from build123d import *

# Parameters (mm, degrees)
SKETCH1_R           = 4
BOSS_EXTRUDE1_DEPTH = 3


with BuildPart() as part:
    # Sketch1 → Boss-Extrude1 (new body)
    with BuildSketch(Plane.XY):
        with BuildLine():
            Line((-3.41129842, 4.305994118), (3.41129842, -4.305994118))
            Line((3.41129842, -4.305994118), (7.005179011, -1.458846897))
            Line((7.005179011, -1.458846897), (8.621253306, -3.498775848))
            Line((8.621253306, -3.498775848), (11.505363509, -2.105535978))
            Line((11.505363509, -2.105535978), (23.000363507, -2.105335353))
            ThreePointArc((23.000363507, -2.105335353), (28.559669511, 3.611172521), (23.925659877, 10.100417487))
            Line((23.925659877, 10.100417487), (0.454659877, 10.100417487))
            Line((0.454659877, 10.100417487), (-0.813143143, 8.410019752))
            Line((-0.813143143, 8.410019752), (0.182582172, 7.153141338))
            Line((0.182582172, 7.153141338), (-3.41129842, 4.305994118))
        make_face()
        with Locations((23.217363507, 3.802664647)):
            Circle(SKETCH1_R, mode=Mode.SUBTRACT)
        Polygon((2.283340507, 4.456152944), (4.860365799, 1.203240304), (2.39128753, -0.752815038), (-0.185737762, 2.500097602), align=None, mode=Mode.SUBTRACT)
    extrude(amount=-BOSS_EXTRUDE1_DEPTH)


solid = part.part
Input: part model. Units: mm. Frame: model coordinates. A direction names the side the tool comes from. Round coordinates to 2 decimals unless told otherwise and drop trailing zeros. Order: outer loops, then holes, each group sorted by start corner. A loop starts at its lowest first (then second) coordinate and runs counter-clockwise, first axis right, second up. Notation, with made-up numbers: (30.25, 36) - (80.25, 36) arc R21 cw to (80.25, 73) - close; hole circle Ø2 at (84, 66). An arc over 180 degrees is marked (long way). Answer as a JSON object with one key per item and string values. Group by question number.
(1) Material intervals for probe 1 along X at (y, z) = (3.5, -2.25); probe 2 along X at (y, z) = (3, -1.75); probe 3 along Y at (x, z) = (0, -0.1), sorted ascending. Write a range as from..to.
(2) Cut plane C-C (z = -1.3). Return loops of the section in (x, y).
(3) Cut plane D-D (x = 17). Return loops of the section in (y, z).
(4) Reachability of faces 5 (the face through (3.554, 2.852, -1.479)), 6 (the face through (-0.17, 9.27, -1.48)), 7 (the face through (-0.32, 7.79, -1.48)), 8 (the face through (7.8, -2.46, -1.48)), 9 (the face through (12, 3, -3)) from +Z, -Z, +X, -X, +Y, -Y: full face, straight path, thin tool, end or side. Return the list, or none.
(5) Draft query along X for faces 1 (the face through (28.55, 3.49, -1.48)), 2 (the face through (0, 0, -1)), 3 (the face through (3.643, 0.239, -1.479)), 4 (the face through (5.183, -2.902, -1.479)). Return one class per face: released by +X, released by -X, zero draft, split by the parting line, or undercut.
(6) Cut plane B-B (y = 6). Return loops of the section in (x, z), then the cut area to 3 significant figures.
(7) Cut plane A-A (x = 1). Return loops of the section in (y, z), then the cut area to 3 significant figures.
(8) Pin query (flat end, axial travel): P1, Ø1, axis at x = 24.5, z = -1, coming from the +Y side. Return the tip coordinate at first contact, or that it passes through.
Here are the results:
{
 "1": {"probe 1": "x = -2.77..1.08, 3.04..19.23, 27.21..28.55", "probe 2": "x = -2.38..0.45, 3.44..19.3, 27.14..28.48", "probe 3": "y = 0..2.27, 2.65..7.01, 7.38..9.49"},
 "2": {"outline": "(-3.41, 4.31) - (3.41, -4.31) - (7.01, -1.46) - (8.62, -3.5) - (11.51, -2.11) - (23, -2.11) arc R6.22 ccw to (23.93, 10.1) - (0.45, 10.1) - (-0.81, 8.41) - (0.18, 7.15) - close; hole (-0.19, 2.5) - (2.39, -0.75) - (4.86, 1.2) - (2.28, 4.46) - close; hole circle Ø8 at (23.22, 3.8)"},
 "3": {"outline": "(-2.11, -3) - (10.1, -3) - (10.1, 0) - (-2.11, 0) - close"},
 "4": {"face 5": "+Z, -Z", "face 6": "+Z, -Z, -X, +Y", "face 7": "+Z, -Z, -X", "face 8": "+Z, -Z, -Y", "face 9": "-Z, +X, -X, +Y, -Y"},
 "5": {"face 1": "released by +X", "face 2": "released by -X", "face 3": "undercut", "face 4": "undercut"},
 "6": {"outline": "(-1.27, -3) - (19.87, -3) - (19.87, 0) - (-1.27, 0) - close; (26.56, -3) - (28.27, -3) - (28.27, 0) - (26.56, 0) - close", "area": "68.6 mm^2"},
 "7": {"outline": "(-1.26, -3) - (1, -3) - (1, 0) - (-1.26, 0) - close; (3.44, -3) - (10.1, -3) - (10.1, 0) - (3.44, 0) - close", "area": "26.8 mm^2"},
 "8": {"P1": "stops at y = 10.08"}
}
